```python
from build123d import *

# Parameters (mm, degrees)
CROQUIS1_W              = 201
CROQUIS1_H              = 201
SALIENTE_EXTRUIR1_DEPTH = 100
VACIADO1_T              = -1


with BuildPart() as part:
    # Croquis1 → Saliente-Extruir1 (new body)
    with BuildSketch(Plane(origin=(0, 0, 0), x_dir=(1, 0, 0), z_dir=(0, 1, 0))):
        with Locations((59.116890843, -76.386715501)):
            Rectangle(CROQUIS1_W, CROQUIS1_H)
    extrude(amount=SALIENTE_EXTRUIR1_DEPTH)

    # Vaciado1
    vaciado1_openings = [part.faces().sort_by_distance(p)[0] for p in [
        (59.116890843, 100, 76.386715501),
    ]]
    offset(amount=VACIADO1_T, openings=vaciado1_openings, kind=Kind.INTERSECTION)


solid = part.part
```
Can you work these out from the model? Positions are in its coordinate system, mm. A direction names the side the tool comes from. Give positions to 0.01 mm unless a question says otherwise; leave off trailing zeros. Order: outer loops, then holes, each group sorted by start corner. A loop starts at its lowest first (then second) coordinate and runs counter-clockwise, first axis right, second up. Notation, with made-up numbers: M 77.25,-6 L 88.25,-6 A22 ccw 88.25,18 Z; hole C 50,77.5 d8. An arc over 180 degrees is marked long. One line per item, written item: value.
1) I want a section at B-B, the plane x = 126. List the corners of the cut face in (y, z) for me, plus the area to 3 significant figures.
Answer sheet:
outline: M 0,-24.11 L 100,-24.11 L 100,-23.11 L 1,-23.11 L 1,175.89 L 100,175.89 L 100,176.89 L 0,176.89 Z
area: 399 mm^2
2) I want a section at C-C, the plane z = 113. List the corners of the cut face in (x, y) for me, plus the area to 3 significant figures.
Answer sheet:
outline: M -41.38,0 L 159.62,0 L 159.62,100 L 158.62,100 L 158.62,1 L -40.38,1 L -40.38,100 L -41.38,100 Z
area: 399 mm^2
3) On a 3-axis mill with a long thin cutter (end or side, diameter ignored), from which of +Z, -Z, +X, -X, +Y, -Y can I reach the whole of each face in a straight line? I mean faces 1 (the face through (58, 50, -23.113)), 2 (the face through (58, 49, -24.113)). Say none if no direction works.
Answer sheet:
face 1: +Y
face 2: -Z, +X, -X, +Y, -Y
4) For P1, Ø6, axis at x = 31, z = 60.5, coming from the +Y side, with a flat end and sliding along its axis, tell me the tip position at first contact or that it passes through.
Answer sheet:
P1: stops at y = 1
5) Please list where these lines run through material, in increasing order: line 1 along Z through (x, y) = (1, 64); line 2 along X through (y, z) = (84.5, -12); line 3 along Y through (x, z) = (128.5, 56.5).
Answer sheet:
line 1: z = -24.11 to -23.11, 175.89 to 176.89
line 2: x = -41.38 to -40.38, 158.62 to 159.62
line 3: y = 0 to 1
6) I want a section at A-A, the plane y = 59. List the corners of the cut face in (x, z) for me, plus the area to 3 significant figures.
Answer sheet:
outline: M -41.38,-24.11 L 159.62,-24.11 L 159.62,176.89 L -41.38,176.89 Z; hole M -40.38,-23.11 L 158.62,-23.11 L 158.62,175.89 L -40.38,175.89 Z
area: 800 mm^2
7) We'd pull the mould along X, two halves only. Please class faces 3 (the face through (58, 49, 176.887)), 4 (the face through (58, 1, 75)), 5 (the face through (158.617, 50, 78)), 6 (the face through (-41.383, 49, 78)): released by +X, released by -X, zero draft, split by the parting line, or undercut.
Answer sheet:
face 3: zero draft
face 4: undercut
face 5: undercut
face 6: released by -X
